Source: three-view drawing plus pictorial views. Frame: mm from the lowest corner of the part. A direction names the side the tool comes from. Give positions to 0.01 mm unless a question says otherwise; leave off trailing zeros. Write each loop counter-clockwise with the first axis right and the second up, starting at its lowest first coordinate (ties: lowest second). Pieces come first, ordered by that corner, then holes. Notation, with made-up numbers: M 55.25,72.25 L 105.25,72.25 A15 ccw 105.25,95.25 Z; hole C 30.5,25 d6. An arc over 180 degrees is marked long. Return JSON: item names as keys, results as strings.
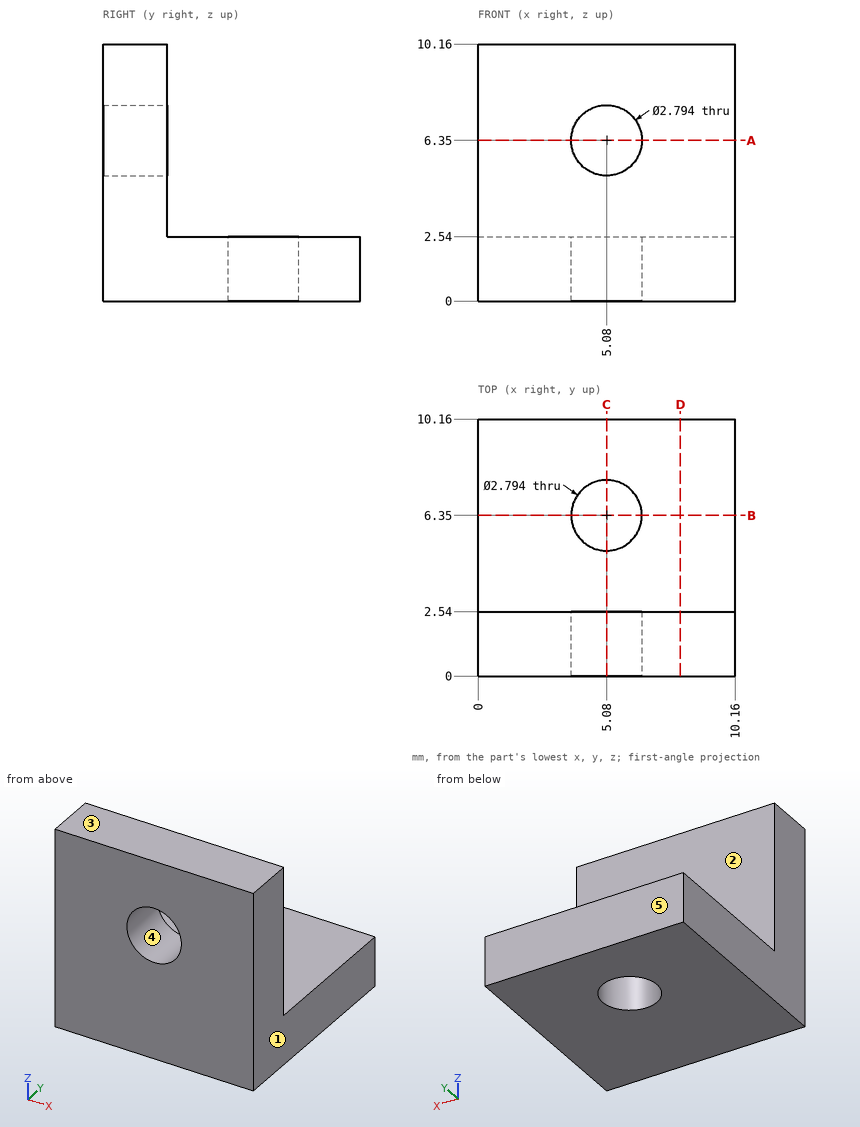
1) Draft query along Z for the marked faces 3, 4 and 5. Return one class per face: released by +Z, released by -Z, zero draft, split by the parting line, or undercut.
Numbers:
{"face 3": "released by +Z", "face 4": "undercut", "face 5": "zero draft"}
2) Line query: line 1 (X direction, y = 1.1, z = 6.35); line 2 (Z direction, x = 5.08, y = 1.05). Output: solid intervals per line, ascending. Write a range as [from, to].
Numbers:
{"line 1": "x = [0, 3.68], [6.48, 10.16]", "line 2": "z = [0, 4.95], [7.75, 10.16]"}
3) Cut plane C-C, the plane x = 5.08. Return the cut outline in (y, z), then the cut area to 3 significant figures.
Numbers:
{"outline": "M 0,0 L 4.95,0 L 4.95,2.54 L 2.54,2.54 L 2.54,4.95 L 0,4.95 Z; M 0,7.75 L 2.54,7.75 L 2.54,10.16 L 0,10.16 Z; M 7.75,0 L 10.16,0 L 10.16,2.54 L 7.75,2.54 Z", "area": "31.0 mm²"}
4) Set-up query: the marked faces 1 and 2. Return all of +Z, -Z, +X, -X, +Y, -Y with unobstructed straight access to the full face (end or side cutting, diameter ignored); none if empty.
Numbers:
{"face 1": "+Z, -Z, +X, +Y, -Y", "face 2": "+Z, +X, -X, +Y"}
5) Contact query for flat-ended pins moving along their axis: pin 1 Ø6 at (x, y) = (6, 6.5) entering from +Z; pin 2 Ø2 at (x, z) = (2.5, 9) entering from +Y. Output: stop coordinate, or through.
Numbers:
{"pin 1": "stops at z = 2.54", "pin 2": "stops at y = 2.54"}
6) Cut plane D-D, the plane x = 8. Return the cut outline in (y, z).
Numbers:
{"outline": "M 0,0 L 10.16,0 L 10.16,2.54 L 2.54,2.54 L 2.54,10.16 L 0,10.16 Z"}
7) Cut plane A-A, the plane z = 6.35. Return the cut outline in (x, y).
Numbers:
{"outline": "M 0,0 L 3.68,0 L 3.68,2.54 L 0,2.54 Z; M 6.48,0 L 10.16,0 L 10.16,2.54 L 6.48,2.54 Z"}
